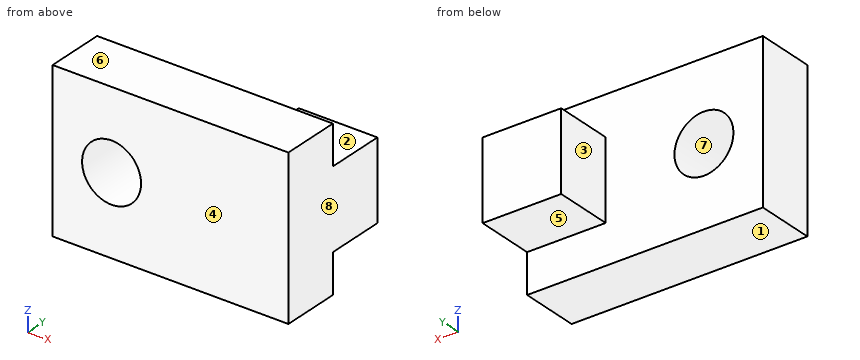
```python
from build123d import *

# Parameters (mm, degrees)
SKETCH1_W           = 60
SKETCH1_H           = 40
BOSS_EXTRUDE1_DEPTH = 15
CUT_EXTRUDE1_REACH  = 17
SKETCH2_R           = 7.5
SKETCH3_W           = 20
SKETCH3_H           = 20
BOSS_EXTRUDE2_DEPTH = 15


with BuildPart() as part:
    # Sketch1 → Boss-Extrude1 (new body)
    with BuildSketch(Plane(origin=(0, 0, 0), x_dir=(1, 0, 0), z_dir=(0, 1, 0))):
        Rectangle(SKETCH1_W, SKETCH1_H)
    extrude(amount=BOSS_EXTRUDE1_DEPTH)

    # Sketch2 → Cut-Extrude1 (cut, up to next)
    with BuildSketch(Plane(origin=(0, 15, 0), x_dir=(1, 0, 0), z_dir=(0, 1, 0)), mode=Mode.PRIVATE) as cut_extrude1_sk1:
        with Locations((-15, 0)):
            Circle(SKETCH2_R)
    cut_extrude1_tool1 = extrude(cut_extrude1_sk1.sketch, amount=-CUT_EXTRUDE1_REACH, mode=Mode.PRIVATE) & part.part
    add(cut_extrude1_tool1.solids().sort_by_distance((-15, 15, 0))[0], mode=Mode.SUBTRACT)

    # Sketch3 → Boss-Extrude2 (add)
    with BuildSketch(Plane(origin=(0, 15, 0), x_dir=(1, 0, 0), z_dir=(0, 1, 0))):
        with Locations((20, 0)):
            Rectangle(SKETCH3_W, SKETCH3_H)
    extrude(amount=BOSS_EXTRUDE2_DEPTH)


solid = part.part
```
Read the model definition and answer for the solid it produces. Units are mm, in the model's axes. Face numbers are marked on the shaded views. A direction names the side the tool comes from. Give positions to 0.01 mm unless a question says otherwise; leave off trailing zeros. Order: outer loops, then holes, each group sorted by start corner. A loop starts at its lowest first (then second) coordinate and runs counter-clockwise, first axis right, second up.
(1) Given pin 1 (12 mm diameter, centred on x = -14.5, y = 24, fed in from -Z); pin 2 (4.5 mm diameter, centred on x = 19.5, y = 22.5, fed in from -Z); pin 3 (4.5 mm diameter, centred on x = 18, y = 24.5, fed in from +Z); pin 4 (12 mm diameter, centred on y = 23, z = 2.5, fed in from -X), each flat-ended and moving along its own axis, determine where each tip first touches the part or whether it passes through.
(2) Find section A-A (z = 0). Give the vertices of the cut face in (x, y).
(3) For the marked faces 1, 2, 3, 4 and 5, determine the directions among +Z, -Z, +X, -X, +Y, -Y from which every point of the face is accessible in a straight line to the end or side of a thin tool.
(4) Find section D-D (x = 14.5). Give the vertices of the cut face in (y, z).
(5) Find section C-C (y = 6.25). Give the vertices of the cut face in (x, z), plus the area to 3 significant figures.
(6) For a pull along Z with two mould halves and no side action, classify the marked faces 6, 7 and 8 as released by +Z, released by -Z, zero draft, split by the parting line, or undercut.
(7) Find section B-B (x = -15). Give the vertices of the cut face in (y, z).
(8) Straight lines are drawn through the part: L1, parallel to X at y = 10.25, z = 0; L2, parallel to Z at x = -15, y = 7.5; L3, parallel to Y at x = -12, z = -13.5. For each, find the intervals that lie inside material, in ascending order.
Result sheet:
1. pin 1: passes through
1. pin 2: stops at z = -10
1. pin 3: stops at z = 10
1. pin 4: stops at x = 10
2. outline: (-30, 0) - (-22.5, 0) - (-22.5, 15) - (-30, 15) - close; (-7.5, 0) - (30, 0) - (30, 30) - (10, 30) - (10, 15) - (-7.5, 15) - close
3. face 1: -Z, +X, -X, +Y, -Y
3. face 2: +Z, +X, -X, +Y
3. face 3: +Z, -Z, -X, +Y
3. face 4: +Z, -Z, +X, -X, -Y
3. face 5: -Z, +X, -X, +Y
4. outline: (0, -20) - (15, -20) - (15, -10) - (30, -10) - (30, 10) - (15, 10) - (15, 20) - (0, 20) - close
5. outline: (-30, -20) - (30, -20) - (30, 20) - (-30, 20) - close; hole circle Ø15 at (-15, 0)
5. area: 2,220 mm2
6. face 6: released by +Z
6. face 7: undercut
6. face 8: zero draft
7. outline: (0, -20) - (15, -20) - (15, -7.5) - (0, -7.5) - close; (0, 7.5) - (15, 7.5) - (15, 20) - (0, 20) - close
8. L1: x = -30 to -22.5, -7.5 to 30
8. L2: z = -20 to -7.5, 7.5 to 20
8. L3: y = 0 to 15
